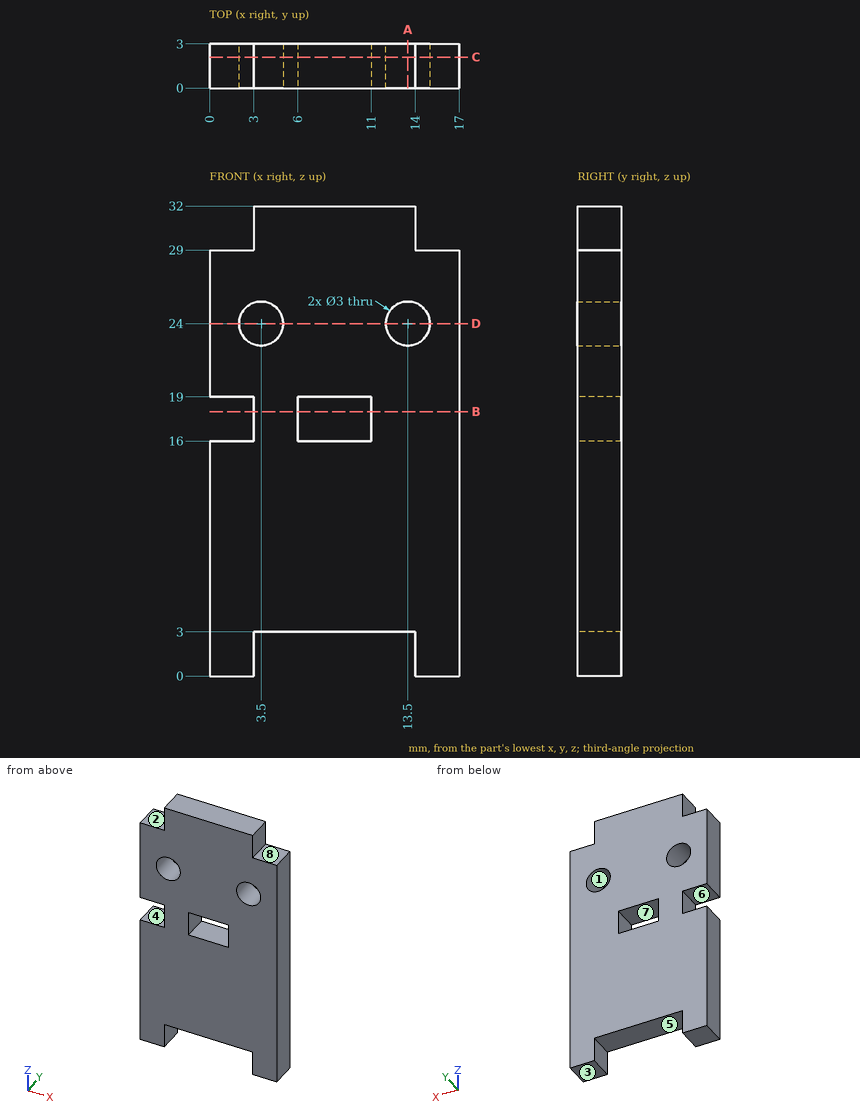
The drawing under review shows one solid part. Ordinate dimensions are in mm from its lowest x, y, z. A direction names the side the tool comes from. Coordinates: 2 decimals unless noted, no trailing zeros. Order: outer loops, then holes, each group sorted by start corner. A loop starts at its lowest first (then second) coordinate and runs counter-clockwise, first axis right, second up. Notation, with made-up numbers: (-29, 88) - (-7, 88) arc R19 cw to (-7, 92) - close; hole circle Ø8 at (9.5, 18). An arc over 180 degrees is marked (long way). Put each result on its own line as item: value.
1) Take a section at C-C, the plane y = 2.1. Give the boundary of the cut face in (x, z).
Response values:
outline: (0, 0) - (3, 0) - (3, 3) - (14, 3) - (14, 0) - (17, 0) - (17, 29) - (14, 29) - (14, 32) - (3, 32) - (3, 29) - (0, 29) - (0, 19) - (3, 19) - (3, 16) - (0, 16) - close; hole circle Ø3 at (3.5, 24); hole (6, 16) - (11, 16) - (11, 19) - (6, 19) - close; hole circle Ø3 at (13.5, 24)
2) Insertion check: P1, Ø1.5, axis at y = 1.5, z = 18, coming from the -X side; P2, Ø0.9, axis at x = 10.5, y = 1, coming from the -Z side; P3, Ø0.9, axis at y = 2, z = 31, coming from the +X side. Each pin has a flat end and moves straight along its axis. Give the tip position at first contact, or say it passes through.
Response values:
P1: stops at x = 3
P2: stops at z = 3
P3: stops at x = 14
3) Take a section at B-B, the plane z = 18. Give the boundary of the cut face in (x, y).
Response values:
outline: (3, 0) - (6, 0) - (6, 3) - (3, 3) - close; (11, 0) - (17, 0) - (17, 3) - (11, 3) - close
4) Tool access review of the marked faces 5, 6, 7 and 8: name each direction out of +Z, -Z, +X, -X, +Y, -Y from which nothing blocks a thin tool from reaching the whole face with its end or side.
Response values:
face 5: -Z, +Y, -Y
face 6: -X, +Y, -Y
face 7: +Y, -Y
face 8: +Z, +X, +Y, -Y
5) The part is to be moulded in two halves that separate along Z. For the marked faces 1, 2, 3 and 4, say which applies: released by +Z, released by -Z, zero draft, split by the parting line, or undercut.
Response values:
face 1: undercut
face 2: released by +Z
face 3: released by -Z
face 4: undercut
6) Take a section at D-D, the plane z = 24. Give the boundary of the cut face in (x, y).
Response values:
outline: (0, 0) - (2, 0) - (2, 3) - (0, 3) - close; (5, 0) - (12, 0) - (12, 3) - (5, 3) - close; (15, 0) - (17, 0) - (17, 3) - (15, 3) - close
7) Wall thickness on L1, parallel to X at y = 1.25, z = 24; L2, parallel to Z at x = 13.5, y = 2; L3, parallel to Z at x = 8, y = 1.25: over which ranges is each line inside the solid? List them lowest first. Write a range as from..to.
Response values:
L1: x = 0..2, 5..12, 15..17
L2: z = 3..22.5, 25.5..32
L3: z = 3..16, 19..32
8) Take a section at A-A, the plane x = 13.5. Give the boundary of the cut face in (y, z), and give its area (3 significant figures).
Response values:
outline: (0, 3) - (3, 3) - (3, 22.5) - (0, 22.5) - close; (0, 25.5) - (3, 25.5) - (3, 32) - (0, 32) - close
area: 78.0 mm²
